from build123d import *

# Parameters (mm, degrees)
SKETCH_1_R      = 1.6
EXTRUDE_1_DEPTH = 3


with BuildPart() as part:
    # 草图1 → 凸台-拉伸1 (new body)
    with BuildSketch(Plane(origin=(0, 0, 0), x_dir=(1, 0, 0), z_dir=(0, 1, 0))):
        Polygon((0, 0), (20, 0), (20, 8), (20, 17.247388719), (12.032168205, 17.247388719), (12.032168205, 8), (0, 8), align=None)
        with Locations(Location((4, 4, 0), (0, 0, 270))):
            Circle(SKETCH_1_R, mode=Mode.SUBTRACT)
        with Locations(Location((13, 4, 0), (0, 0, 270))):
            Circle(SKETCH_1_R, mode=Mode.SUBTRACT)
        with Locations(Location((16.016084103, 13.971325548, 0), (0, 0, 270))):
            Circle(SKETCH_1_R, mode=Mode.SUBTRACT)
    extrude(amount=EXTRUDE_1_DEPTH)


solid = part.part
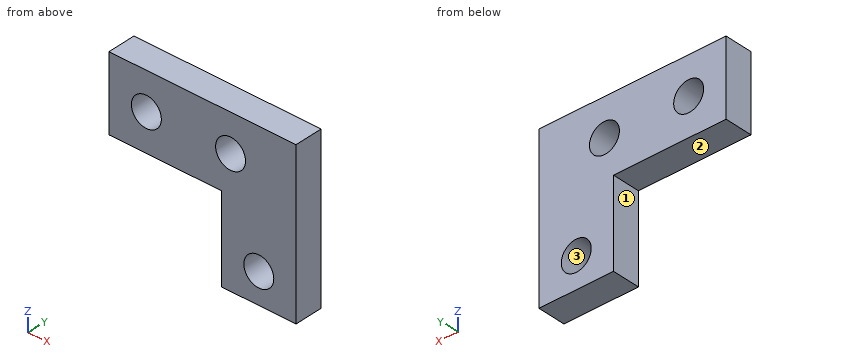
Verification items for the finished model (mm, model axes). Face numbers are marked on the shaded views. Give positions to 0.01 mm unless a question says otherwise; leave off trailing zeros. Order: outer loops, then holes, each group sorted by start corner. A loop starts at its lowest first (then second) coordinate and runs counter-clockwise, first axis right, second up. Notation, with made-up numbers: M 82,23.25 L 137,23.25 A12 cw 137,39.25 Z; hole C 77.25,20 d4. An arc over 180 degrees is marked long. Answer as a JSON object with one key per item and string values. Group by question number.
1) Mould release check, pull along X, two halves, no side actions. Record for the marked faces 1, 2 and 3: released by +X, released by -X, zero draft, split by the parting line, or undercut.
2) Cross-section at B-B (x = 4). Enter the section's corners in (y, z).
3) Depth check by flat-ended pin: pin 1 Ø0.9 at (x, y) = (7.5, 1.5) entering from -Z; pin 2 Ø1.5 at (y, z) = (1.5, -14.5) entering from -X. Enter the tip coordinate at first touch or a pass-through.
4) Cross-section at C-C (y = 0.5). Enter the section's corners in (x, z), then the cut area to 3 significant figures.
5) Cross-section at D-D (z = -14.25). Enter the section's corners in (x, y).
6) Scan lines: line 1 along X through (y, z) = (0.75, -4); line 2 along Z through (x, y) = (9, 2.25); line 3 along Z through (x, y) = (12.5, 0.5). Record each from-to range of solid material in increasing order. Write a range as [from, to].
7) Cross-section at A-A (z = -4). Enter the section's corners in (x, y).
Result sheet:
{
 "1": {"face 1": "released by -X", "face 2": "zero draft", "face 3": "undercut"},
 "2": {"outline": "M 0,-8 L 3,-8 L 3,-5.6 L 0,-5.6 Z; M 0,-2.4 L 3,-2.4 L 3,0 L 0,0 Z"},
 "3": {"pin 1": "stops at z = -8", "pin 2": "stops at x = 12.03"},
 "4": {"outline": "M 0,-8 L 12.03,-8 L 12.03,-17.25 L 20,-17.25 L 20,0 L 0,0 Z; hole C 4,-4 d3.2; hole C 13,-4 d3.2; hole C 16.02,-13.97 d3.2", "area": "210 mm2"},
 "5": {"outline": "M 12.03,0 L 14.44,0 L 14.44,3 L 12.03,3 Z; M 17.59,0 L 20,0 L 20,3 L 17.59,3 Z"},
 "6": {"line 1": "x = [0, 2.4], [5.6, 11.4], [14.6, 20]", "line 2": "z = [-8, 0]", "line 3": "z = [-17.25, -5.52], [-2.48, 0]"},
 "7": {"outline": "M 0,0 L 2.4,0 L 2.4,3 L 0,3 Z; M 5.6,0 L 11.4,0 L 11.4,3 L 5.6,3 Z; M 14.6,0 L 20,0 L 20,3 L 14.6,3 Z"}
}
